```python
from build123d import *

# Parameters (mm, degrees)
SKETCH1_W                            = 139.7
SKETCH1_H                            = 102.87
BOSS_EXTRUDE1_DEPTH                  = 19.05
F_10_32_TAPPED_HOLE2_D               = 4.0386
F_10_32_TAPPED_HOLE2_DEPTH           = 13.716
F_10_32_TAPPED_HOLE2_TIP             = 1.213317848
F_10_32_TAPPED_HOLE2_ON_FACE_2_D     = 4.0386
F_10_32_TAPPED_HOLE2_ON_FACE_2_DEPTH = 13.716
F_10_32_TAPPED_HOLE2_ON_FACE_2_TIP   = 1.213317848


with BuildPart() as part:
    # Sketch1 → Boss-Extrude1 (new body)
    with BuildSketch(Plane.XY):
        with Locations((69.85, 51.435)):
            Rectangle(SKETCH1_W, SKETCH1_H)
        Polygon((19.05, 19.05), (19.05, 73.152), (92.075, 19.05), align=None, mode=Mode.SUBTRACT)
        Polygon((120.65, 83.82), (120.65, 29.718), (47.625, 83.82), align=None, mode=Mode.SUBTRACT)
    extrude(amount=BOSS_EXTRUDE1_DEPTH)

    # #10-32 Tapped Hole2
    with Locations(Plane(origin=(0, 77.63256, 6.35), x_dir=(0, 0, -1), z_dir=(-1, 0, 0))):
        with Locations((0, 0), (0, 67.31)):
            Hole(F_10_32_TAPPED_HOLE2_D / 2, depth=F_10_32_TAPPED_HOLE2_DEPTH)
            with Locations((0, 0, -(F_10_32_TAPPED_HOLE2_DEPTH + F_10_32_TAPPED_HOLE2_TIP / 2))):  # 118° drill point
                Cone(0, F_10_32_TAPPED_HOLE2_D / 2, F_10_32_TAPPED_HOLE2_TIP, mode=Mode.SUBTRACT)

    # #10-32 Tapped Hole2 on face 2
    with Locations(Plane(origin=(139.7, 10.32256, 6.35), x_dir=(0, 0, 1), z_dir=(1, 0, 0))):
        with Locations((0, 0), (0, -67.31)):
            Hole(F_10_32_TAPPED_HOLE2_ON_FACE_2_D / 2, depth=F_10_32_TAPPED_HOLE2_ON_FACE_2_DEPTH)
            with Locations((0, 0, -(F_10_32_TAPPED_HOLE2_ON_FACE_2_DEPTH + F_10_32_TAPPED_HOLE2_ON_FACE_2_TIP / 2))):  # 118° drill point
                Cone(0, F_10_32_TAPPED_HOLE2_ON_FACE_2_D / 2, F_10_32_TAPPED_HOLE2_ON_FACE_2_TIP, mode=Mode.SUBTRACT)


solid = part.part
```
Work out the finished part from the listing and answer in its coordinate system (mm). A direction names the side the tool comes from. Round coordinates to 2 decimals unless told otherwise and drop trailing zeros. Loops run counter-clockwise (first coordinate to the right, second up) from the corner with the lowest first, then second, coordinate; pieces in that order, holes last. Notation, with made-up numbers: (-13.75, 14.5) -> (39.25, 14.5) arc R17 cw to (39.25, 34.5) -> close; hole circle Ø10 at (5.5, -14). An arc over 180 degrees is marked (long way). Write each question's results on one line, items separated by ' | '. Start each with the question number.
1. Section B-B (z = 15) is taken. Determine the outline of the cut face in (x, y) (3 decimals).
2. Section A-A (y = 46.5) is taken. Determine the outline of the cut face in (x, z), plus the area to 3 significant figures.
3. Given pin 1 Ø8 at (y, z) = (46.5, 2.5) entering from -X; pin 2 Ø2.5 at (y, z) = (10.32, 6.35) entering from +X, each flat-ended and moving along its own axis, determine where each tip first touches the part or whether it passes through.
4. A tool of negligible diameter and unlimited length cuts with its end or side. For faces 1 (the face through (132.746, 11.096, 4.485)), 2 (the face through (6.954, 12.294, 5.912)), 3 (the face through (55.05, 46.48, 9.39)), 4 (the face through (69, 102.87, 9)), 5 (the face through (0, 51, 9)), from which of +Z, -Z, +X, -X, +Y, -Y can it reach the whole face along a straight path? Write none if from no direction.
5. For a pull along Z with two mould halves and no side action, classify faces 6 (the face through (139.7, 51, 9)), 7 (the face through (69, 52, 19.05)), 8 (the face through (14.719, 9.975, 6.396)) as +Z half, -Z half, draft (parallel to the pull), parting line (faces both ways), or undercut.
6. Find the intervals of material crossed by probe 1 along Y at (x, z) = (131.5, 6.35); probe 2 along Y at (x, z) = (51, 9); probe 3 along X at (y, z) = (65, 16), in increasing order. Write a range as from..to.
Evaluation:
1) outline: (0, 0) -> (139.7, 0) -> (139.7, 102.87) -> (0, 102.87) -> close; hole (19.05, 19.05) -> (92.075, 19.05) -> (19.05, 73.152) -> close; hole (47.625, 83.82) -> (120.65, 29.718) -> (120.65, 83.82) -> close
2) outline: (0, 0) -> (19.05, 0) -> (19.05, 19.05) -> (0, 19.05) -> close; (55.02, 0) -> (98, 0) -> (98, 19.05) -> (55.02, 19.05) -> close; (120.65, 0) -> (139.7, 0) -> (139.7, 19.05) -> (120.65, 19.05) -> close | area: 1,540 mm2
3) pin 1: stops at x = 0 | pin 2: stops at x = 125.52
4) face 1: +X | face 2: -X | face 3: +Z, -Z | face 4: +Z, -Z, +X, -X, +Y | face 5: +Z, -Z, -X, +Y, -Y
5) face 6: draft | face 7: +Z half | face 8: undercut
6) probe 1: y = 0..8.3, 12.34..75.61, 79.65..102.87 | probe 2: y = 0..19.05, 49.48..81.32, 83.82..102.87 | probe 3: x = 0..19.05, 30.05..73.03, 120.65..139.7
